Input: part model. Units: mm. Frame: model coordinates. Face numbers are marked on the shaded views. A direction names the side the tool comes from. Coordinates: 2 decimals unless noted, no trailing zeros. Order: outer loops, then holes, each group sorted by start corner. A loop starts at its lowest first (then second) coordinate and runs counter-clockwise, first axis right, second up. Notation, with made-up numbers: M -27,-29 L 24,-29 A24 cw 24,7 Z; hole C 39.5,81.25 d3. An arc over 180 degrees is marked long. One line per item, written item: value.
```python
from build123d import *

# Parameters (mm, degrees)
F0_R     = 6
F1_DEPTH = 3
F3_DEPTH = 3
F5_D     = 4.1


with BuildPart() as f1:
    # F0 (on Right) → F1 (new body)
    with BuildSketch(Plane.YZ):
        Circle(F0_R)
    extrude(amount=F1_DEPTH)

    # F2 (on face) → F3 (join)
    with BuildSketch(Plane.YZ.offset(3)):
        Polygon((4.9074772881, 8.5), (-4.9074772881, 8.5), (-9.8149545762, 0), (-4.9074772881, -8.5), (4.9074772881, -8.5), (9.8149545762, 0), align=None)
    extrude(amount=F3_DEPTH)

    # F5 (through all)
    with Locations(Plane.YZ.offset(6)):
        with Locations((0, 0)):
            Hole(F5_D / 2)


solid = f1.part
```
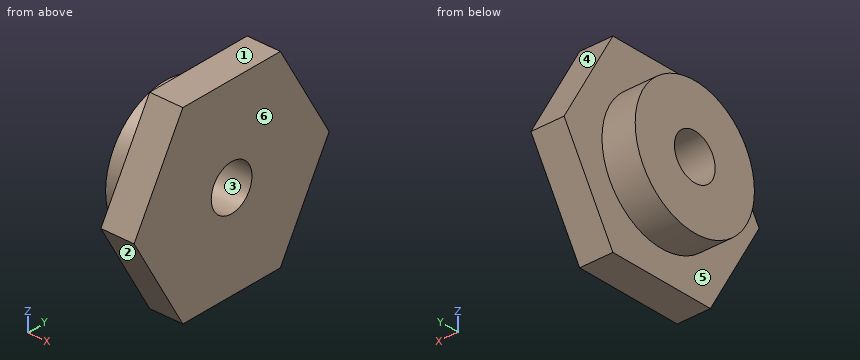
(1) Cut plane D-D on z = 2.5. Output: boundary loops of the cut face in (x, y).
Data:
outline: M 0,-5.45 L 3,-5.45 L 3,-8.37 L 6,-8.37 L 6,8.37 L 3,8.37 L 3,5.45 L 0,5.45 Z
(2) Ray query, line 1 (Z direction, x = 2, y = 0); line 2 (Z direction, x = 3.55, y = 0); line 3 (X direction, y = 6.75, z = -1.5). Return the intervals inside material, ascending. Write a range as from..to.
Data:
line 1: z = -6..-2.05, 2.05..6
line 2: z = -8.5..-2.05, 2.05..8.5
line 3: x = 3..6
(3) Access query for the marked faces 5 and 6. Directions: +Z, -Z, +X, -X, +Y, -Y. A direction counts if a zero-diameter tool reaches every point of the face in a straight line with its end or side. Return the directions, or none.
Data:
face 5: -X
face 6: +Z, -Z, +X, +Y, -Y
(4) Draft query along Y for the marked faces 1, 2, 3 and 4. Return one class per face: released by +Y, released by -Y, zero draft, split by the parting line, or undercut.
Data:
face 1: zero draft
face 2: released by -Y
face 3: undercut
face 4: released by +Y
(5) Cut plane A-A on y = 0. Output: boundary loops of the cut face in (x, z).
Data:
outline: M 0,-6 L 3,-6 L 3,-8.5 L 6,-8.5 L 6,-2.05 L 0,-2.05 Z; M 0,2.05 L 6,2.05 L 6,8.5 L 3,8.5 L 3,6 L 0,6 Z
(6) Cut plane C-C on z = -0.25. Output: boundary loops of the cut face in (x, y).
Data:
outline: M 0,-5.99 L 3,-5.99 L 3,-9.67 L 6,-9.67 L 6,-2.03 L 0,-2.03 Z; M 0,2.03 L 6,2.03 L 6,9.67 L 3,9.67 L 3,5.99 L 0,5.99 Z
(7) First-contact query: pin 1 (8 mm diameter, centred on y = -3.5, z = -3, fed in from -X); pin 2 (1.5 mm diameter, centred on x = 3, z = -1, fed in from +Y); pin 3 (2 mm diameter, centred on x = 3, z = -4, fed in from +Y). Flat tips, straight axial feed; report the tip coordinate or a pass-through.
Data:
pin 1: stops at x = 0
pin 2: stops at y = 9.67
pin 3: stops at y = 8.08
(8) Cut plane B-B on x = 5.55. Output: boundary loops of the cut face in (y, z), plus the area to 3 significant figures.
Data:
outline: M -9.81,0 L -4.91,-8.5 L 4.91,-8.5 L 9.81,0 L 4.91,8.5 L -4.91,8.5 Z; hole C 0,0 d4.1
area: 237 mm2
